```python
from build123d import *

# Parameters (mm, degrees)
CYLINDER023_R             = 3
CYLINDER023_DEPTH         = 60
CYLINDER023_PITCH_ANGLE   = 90
CYLINDER022_R             = 3
CYLINDER022_DEPTH         = 100
CYLINDER022_ROLL_ANGLE    = 90
CYLINDER024_R             = 3
CYLINDER024_DEPTH         = 60
CYLINDER024_PITCH_ANGLE   = 90
FUSION009_PLACEMENT_ANGLE = 180


with BuildPart() as cylinder029:
    # Cylinder023 → Cylinder023 (new body)
    with BuildSketch(Plane.XY):
        Circle(CYLINDER023_R)
    extrude(amount=CYLINDER023_DEPTH)


with BuildPart() as cylinder029_1:
    # Cylinder023 pitch: moved
    add(cylinder029.part.rotate(Axis((0, 0, 0), (0, 1, 0)), CYLINDER023_PITCH_ANGLE))


with BuildPart() as cylinder029_2:
    # Cylinder023 placement: moved
    add(cylinder029_1.part.moved(Location((-50, -3, 0))))


with BuildPart() as fusion008:
    # Cylinder022 → Cylinder022 (new body)
    with BuildSketch(Plane.XY):
        Circle(CYLINDER022_R)
    extrude(amount=CYLINDER022_DEPTH)


with BuildPart() as fusion008_1:
    # Cylinder022 roll: moved
    add(fusion008.part.rotate(Axis((0, 0, 0), (1, 0, 0)), CYLINDER022_ROLL_ANGLE))


with BuildPart() as fusion008_2:
    # Cylinder022 placement: moved
    add(fusion008_1.part.moved(Location((-50, 0, 0))))

    # Fusion008: union Cylinder029
    add(cylinder029_2.part)


with BuildPart() as handle_right:
    # Cylinder024 → Cylinder024 (new body)
    with BuildSketch(Plane.XY):
        Circle(CYLINDER024_R)
    extrude(amount=CYLINDER024_DEPTH)


with BuildPart() as handle_right_1:
    # Cylinder024 pitch: moved
    add(handle_right.part.rotate(Axis((0, 0, 0), (0, 1, 0)), CYLINDER024_PITCH_ANGLE))


with BuildPart() as handle_right_2:
    # Cylinder024 placement: moved
    add(handle_right_1.part.moved(Location((-50, -97, 0))))

    # Fusion009: union Fusion008
    add(fusion008_2.part)


with BuildPart() as handle_right_3:
    # Fusion009 placement: moved
    add(handle_right_2.part.moved(Location((500, 165, 230))).rotate(Axis((500, 165, 230), (0, 1, 0)), FUSION009_PLACEMENT_ANGLE))


solid = handle_right_3.part
```
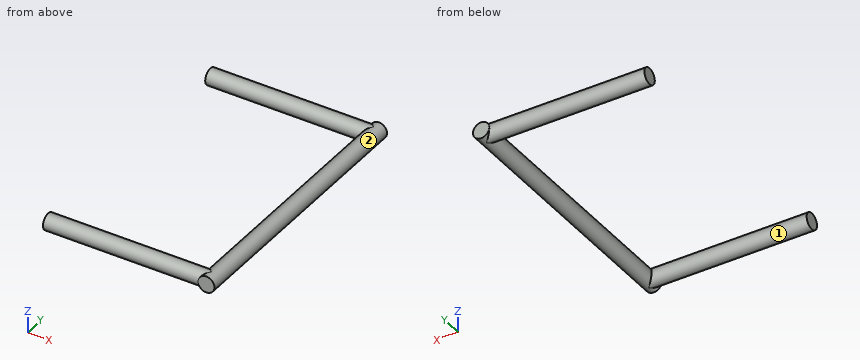
Check sheet for the modelled part. Datum: model origin and axes. Units: mm. Face numbers are marked on the shaded views. A direction names the side the tool comes from. Coordinates: 2 decimals unless noted, no trailing zeros. Loops run counter-clockwise (first coordinate to the right, second up) from the corner with the lowest first, then second, coordinate; pieces in that order, holes last.
1) Sectioned sample at D-D (x = 548.5). Record the boundary of the cut face in (y, z), and give its area (3 significant figures).
2) Gauge pin test, flat end, axial feed: pin 1 (2 mm diameter, centred on x = 514.5, z = 231.5, fed in from -Y). Record the tip position at first contact, or that the pin passes through.
3) Material ranges on probe 1 along Y at (x, z) = (513, 230.2); probe 2 along X at (y, z) = (106, 229.9); probe 3 along Y at (x, z) = (544.5, 232), recorded low to high.
4) Sectioned sample at C-C (z = 229). Record the boundary of the cut face in (x, y), and give its area (3 significant figures).
5) Access from +Z, -Z, +X, -X, +Y, -Y to the whole of each face (thin tool, end or side, straight path). Record for the marked faces 1 and 2.
6) Sectioned sample at A-A (x = 536). Record the boundary of the cut face in (y, z), and give its area (3 significant figures).
7) Sectioned sample at B-B (y = 131.5). Record the boundary of the cut face in (x, z).
Check sheet entries:
1. outline: (65, 227.4) - (66.5, 227.4) arc R3 ccw to (69.5, 227.4) - (160.5, 227.4) arc R3 ccw to (163.5, 227.4) - (165, 227.4) - (165, 232.6) - (163.5, 232.6) arc R3 ccw to (160.5, 232.6) - (69.5, 232.6) arc R3 ccw to (66.5, 232.6) - (65, 232.6) - close
1. area: 523 mm2
2. pin 1: stops at y = 65.04
3. probe 1: y = 65.01 to 70.99, 159.01 to 164.99
3. probe 2: x = 547 to 553
3. probe 3: y = 65.76 to 70.24, 159.76 to 164.24
4. outline: (490, 65.17) - (547.17, 65.17) - (547.17, 65) - (552.83, 65) - (552.83, 165) - (547.17, 165) - (547.17, 164.83) - (490, 164.83) - (490, 159.17) - (547.17, 159.17) - (547.17, 70.83) - (490, 70.83) - close
4. area: 1,210 mm2
5. face 1: -X
5. face 2: none
6. outline: circle Ø6 at (68, 230); circle Ø6 at (162, 230)
6. area: 56.5 mm2
7. outline: circle Ø6 at (550, 230)
